```python
from build123d import *

# Parameters (mm, degrees)
F0_W     = 15
F0_H     = 15
F0_R     = 2.25
F1_DEPTH = 2.5
F2_W     = 15
F2_H     = 20
F2_R     = 2.25
F3_DEPTH = 5
F4_W     = 15
F4_H     = 20
F4_R     = 2.5
F5_DEPTH = 9


with BuildPart() as f1:
    # F0 (on Top) → F1 (new body)
    with BuildSketch(Plane.XY):
        with Locations((7.5, 7.5)):
            Rectangle(F0_W, F0_H)
        with Locations((7.5, 10.905)):
            Circle(F0_R, mode=Mode.SUBTRACT)
    extrude(amount=F1_DEPTH)

    # F2 (on face) → F3 (join)
    with BuildSketch(Plane.XY.offset(2.5)):
        with Locations((7.5, 5)):
            Rectangle(F2_W, F2_H)
        with Locations((7.5, 10.905)):
            Circle(F2_R, mode=Mode.SUBTRACT)
    extrude(amount=F3_DEPTH)

    # F4 (on face) → F5 (join)
    with BuildSketch(Plane(origin=(0, 0, 0), x_dir=(1, 0, 0), z_dir=(0, 0, -1))):
        with Locations((7.5, -5)):
            Rectangle(F4_W, F4_H)
        with Locations((7.5, -10.905)):
            Circle(F4_R, mode=Mode.SUBTRACT)
    extrude(amount=F5_DEPTH)


solid = f1.part
```
Here's how the part is built. I have some questions about the finished solid (model axes, mm). A direction names the side the tool comes from. Coordinates: 2 decimals unless noted, no trailing zeros. Loops run counter-clockwise (first coordinate to the right, second up) from the corner with the lowest first, then second, coordinate; pieces in that order, holes last. Notation, with made-up numbers: (9, 58) -> (28, 58) arc R17 ccw to (28, 82) -> close; hole circle Ø7 at (81, 38). An arc over 180 degrees is marked (long way). Return JSON: item names as keys, results as strings.
1) If we section it at A-A, the plane x = 7.5: Write out the boundary of the cut face in (y, z) (3 decimals), then the cut area to 3 significant figures.
Results below:
{"outline": "(-5, -9) -> (8.405, -9) -> (8.405, 0) -> (8.655, 0) -> (8.655, 7.5) -> (-5, 7.5) -> (-5, 2.5) -> (0, 2.5) -> (0, 0) -> (-5, 0) -> close; (13.155, 0) -> (13.405, 0) -> (13.405, -9) -> (15, -9) -> (15, 7.5) -> (13.155, 7.5) -> close", "area": "239 mm²"}
2) I need wall thicknesses on line 1 (Y direction, x = 7.5, z = 6) (3 decimals); line 2 (X direction, y = 11, z = -7.75); line 3 (Z direction, x = 3.5, y = -1.25). Which ranges of each line are inside material? Lowest first, please. Write a range as from..to.
Results below:
{"line 1": "-5..8.655, 13.155..15", "line 2": "0..5, 10..15", "line 3": "-9..0, 2.5..7.5"}
3) If we section it at C-C, the plane z = -6.25: Write out the boundary of the cut face in (x, y) (3 decimals).
Results below:
{"outline": "(0, -5) -> (15, -5) -> (15, 15) -> (0, 15) -> close; hole circle Ø5 at (7.5, 10.905)"}
4) For faces 1 (the face through (7, 15, -1)), 2 (the face through (7, -2, 2.5)), 3 (the face through (9.9, 10.2, -4.4)), which set-ups out of +Z, -Z, +X, -X, +Y, -Y let a thin tool reach every point of the face, with its end or its side?
Results below:
{"face 1": "+Z, -Z, +X, -X, +Y", "face 2": "+X, -X, -Y", "face 3": "-Z"}
5) If we section it at D-D, the plane x = 11.25: Write out the boundary of the cut face in (y, z).
Results below:
{"outline": "(-5, -9) -> (15, -9) -> (15, 7.5) -> (-5, 7.5) -> (-5, 2.5) -> (0, 2.5) -> (0, 0) -> (-5, 0) -> close"}
6) Will these pins go through, and if not, where does the flat tip stop? pin 1 (2.5 mm diameter, centred on x = 7.5, y = 10.905, fed in from +Z); pin 2 (0.8 mm diameter, centred on x = 4, z = 1, fed in from -Y).
Results below:
{"pin 1": "through", "pin 2": "y = 0"}
7) Thinking about a two-plate mould opening in Z: for faces 4 (the face through (7.207, 13.136, 3.698)), 5 (the face through (7, 0, 1)), 6 (the face through (7, 5, -9)), which applies, +Z half, -Z half, draft (parallel to the pull), parting line (faces both ways), or undercut?
Results below:
{"face 4": "draft", "face 5": "undercut", "face 6": "-Z half"}
8) If we section it at B-B, the plane y = -0.25: Write out the boundary of the cut face in (x, z), then the cut area to 3 significant figures.
Results below:
{"outline": "(0, -9) -> (15, -9) -> (15, 0) -> (0, 0) -> close; (0, 2.5) -> (15, 2.5) -> (15, 7.5) -> (0, 7.5) -> close", "area": "210 mm²"}
